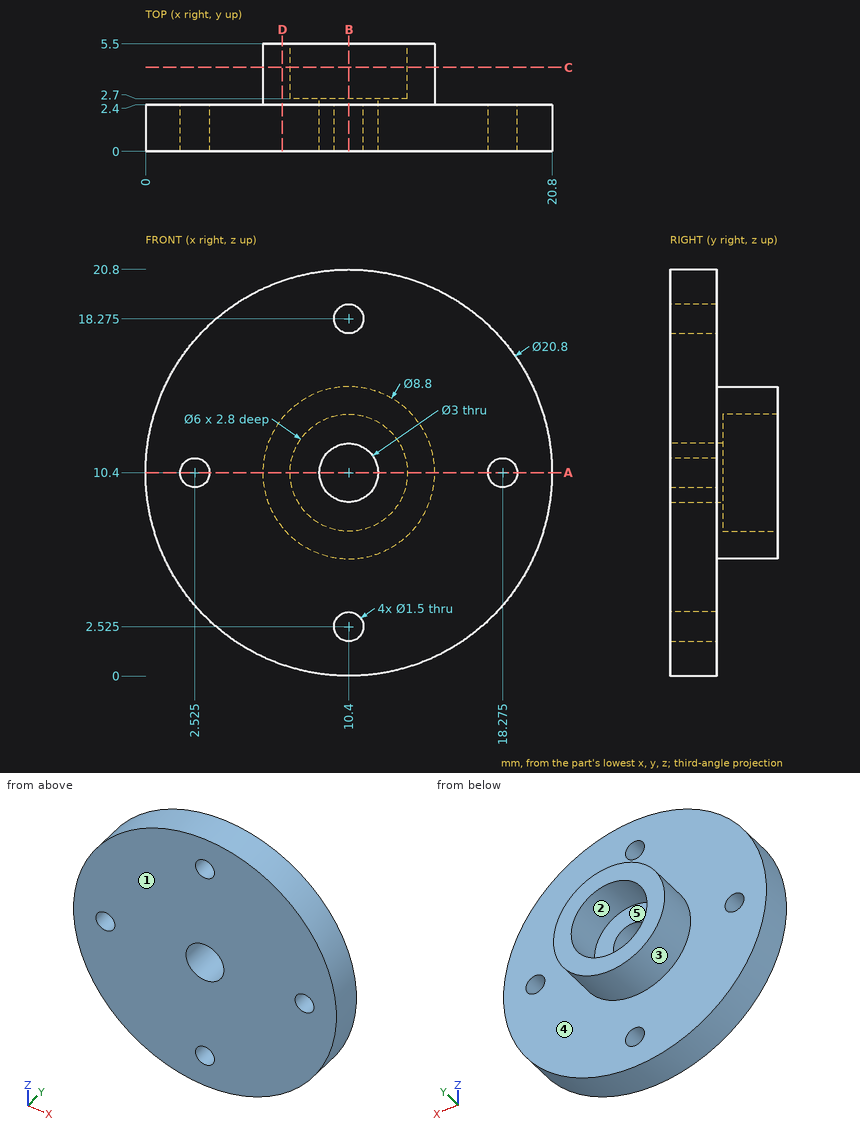
The drawing under review shows one solid part. Ordinate dimensions are in mm from its lowest x, y, z. A direction names the side the tool comes from. Round coordinates to 2 decimals unless told otherwise and drop trailing zeros. Write each loop counter-clockwise with the first axis right and the second up, starting at its lowest first coordinate (ties: lowest second). Pieces come first, ordered by that corner, then holes. Notation, with made-up numbers: (14, 76.5) - (41, 76.5) arc R20 ccw to (41, 114.5) - close; hole circle Ø5 at (67.25, 66). An arc over 180 degrees is marked (long way). Put each result on its own line as item: value.
Q1. Mouldability with a two-part tool opening along X and no side actions: class the marked faces 3, 4 and 5 as released by +X, released by -X, zero draft, split by the parting line, or undercut.
Solved:
face 3: split by the parting line
face 4: zero draft
face 5: undercut
Q2. We need section D-D (x = 7). Give the boundary of the cut face in (y, z), and give its area (3 significant figures).
Solved:
outline: (0, 0.57) - (2.4, 0.57) - (2.4, 7.61) - (5.5, 7.61) - (5.5, 13.19) - (2.4, 13.19) - (2.4, 20.23) - (0, 20.23) - close
area: 64.5 mm2
Q3. We need section B-B (x = 10.4). Give the boundary of the cut face in (y, z) (3 decimals).
Solved:
outline: (0, 0) - (2.4, 0) - (2.4, 1.775) - (0, 1.775) - close; (0, 3.275) - (2.4, 3.275) - (2.4, 6) - (5.5, 6) - (5.5, 7.4) - (2.7, 7.4) - (2.7, 8.9) - (0, 8.9) - close; (0, 11.9) - (2.7, 11.9) - (2.7, 13.4) - (5.5, 13.4) - (5.5, 14.8) - (2.4, 14.8) - (2.4, 17.525) - (0, 17.525) - close; (0, 19.025) - (2.4, 19.025) - (2.4, 20.8) - (0, 20.8) - close
Q4. Wall thickness on probe 1 along X at (y, z) = (0.7, 10.4) (3 decimals); probe 2 along Y at (x, z) = (8, 3.75); probe 3 along X at (y, z) = (4.2, 10.4): over which ranges is each line inside the solid? List them lowest first.
Solved:
probe 1: x = 0 to 1.775, 3.275 to 8.9, 11.9 to 17.525, 19.025 to 20.8
probe 2: y = 0 to 2.4
probe 3: x = 6 to 7.4, 13.4 to 14.8
Q5. Insertion check: pin 1 Ø3 at (x, y) = (7.5, 1) entering from -Z; pin 2 Ø2 at (x, z) = (18.275, 10.4) entering from +Y; pin 3 Ø1.8 at (x, z) = (10.4, 10.4) entering from -Y; pin 4 Ø1 at (x, y) = (14, 1.5) entering from +Z. Each pin has a flat end and moves straight along its axis. Give the tip position at first contact, or say it passes through.
Solved:
pin 1: stops at z = 0.09
pin 2: stops at y = 2.4
pin 3: passes through
pin 4: stops at z = 20.33
Q6. Machinability: for the marked faces 1 and 2, which of the approach directions +Z, -Z, +X, -X, +Y, -Y give a long, thin tool a straight path to every point of the face, cutting with its end or side? Answer none if there is none.
Solved:
face 1: +Z, -Z, +X, -X, -Y
face 2: +Y
Q7. We need section C-C (y = 4.3). Give the boundary of the cut face in (x, z), and give its area (3 significant figures).
Solved:
outline: circle Ø8.8 at (10.4, 10.4); hole circle Ø6 at (10.4, 10.4)
area: 32.5 mm2
Q8. We need section A-A (z = 10.4). Give the boundary of the cut face in (x, y) (3 decimals).
Solved:
outline: (0, 0) - (1.775, 0) - (1.775, 2.4) - (0, 2.4) - close; (3.275, 0) - (8.9, 0) - (8.9, 2.7) - (7.4, 2.7) - (7.4, 5.5) - (6, 5.5) - (6, 2.4) - (3.275, 2.4) - close; (11.9, 0) - (17.525, 0) - (17.525, 2.4) - (14.8, 2.4) - (14.8, 5.5) - (13.4, 5.5) - (13.4, 2.7) - (11.9, 2.7) - close; (19.025, 0) - (20.8, 0) - (20.8, 2.4) - (19.025, 2.4) - close
